```python
from build123d import *

# Parameters (mm, degrees)
SKETCH_1_R      = 3
EXTRUDE_1_DEPTH = 14
CHAMFER_1_SIZE  = 0.1


with BuildPart() as part:
    # 草图1 → 凸台-拉伸1 (new, symmetric)
    with BuildSketch(Plane(origin=(0, 0, 0), x_dir=(1, 0, 0), z_dir=(0, 1, 0))):
        with Locations(Location((0, 0, 0), (0, 0, 270))):
            Circle(SKETCH_1_R)
    extrude(amount=EXTRUDE_1_DEPTH, both=True)

    # 草图3 → M4 Tapped Hole1 (revolve, cut)
    with BuildSketch(Plane(origin=(0, 14, 0), x_dir=(0, 0, 1), z_dir=(1, 0, 0))):
        Polygon((0, 0), (0, 28), (1.675, 28), (1.65, 27.975), (1.65, 0.375), (2.025, 0), align=None)
    revolve(axis=Axis((0, 20.35, 0), (0, -1, 0)), mode=Mode.SUBTRACT)

    # 倒角1
    chamfer_1_edges = [part.edges().sort_by_distance(p)[0] for p in [
        (0, -14, -3),
        (0, 14, -3),
    ]]
    chamfer(chamfer_1_edges, length=CHAMFER_1_SIZE)


solid = part.part
```
Can you work these out from the model? Positions are in its coordinate system, mm. Give positions to 0.01 mm unless a question says otherwise; leave off trailing zeros. Write each loop counter-clockwise with the first axis right and the second up, starting at its lowest first coordinate (ties: lowest second). Pieces come first, ordered by that corner, then holes. Notation, with made-up numbers: (-27, 26) -> (20, 26) arc R21 cw to (20, 45) -> close; hole circle Ø6 at (66.25, 21.25). An arc over 180 degrees is marked (long way). Write item = value, one per line.
(1) I need wall thicknesses on probe 1 along X at (y, z) = (-2.25, 0); probe 2 along Z at (x, y) = (-0.65, -4); probe 3 along X at (y, z) = (7.75, 1.05). Which ranges of each line are inside material? Lowest first, please. Write a range as from..to.
Worked out:
probe_1 = -3..-1.65, 1.65..3
probe_2 = -2.93..-1.52, 1.52..2.93
probe_3 = -2.81..-1.27, 1.27..2.81
(2) I'm going to push flat-ended pins straight in: P1, Ø1.5, axis at y = 3.5, z = -1, coming from the -X side; P2, Ø3, axis at x = 0, z = 0.5, coming from the +Y side (3 decimals); P3, Ø3, axis at x = -2, y = 6, coming from the -Z side. Where does each tip first touch, or does it pass through?
Worked out:
P1 = -2.99
P2 = 13.975
P3 = -2.96
(3) Suppose I cut it at A-A on z = 0. Write out the boundary of the cut face in (x, y) (3 decimals), then the cut area to 3 significant figures.
Worked out:
outline = (-3, -13.9) -> (-2.9, -14) -> (-1.675, -14) -> (-1.65, -13.975) -> (-1.65, 13.625) -> (-2.025, 14) -> (-2.9, 14) -> (-3, 13.9) -> close; (1.65, -13.975) -> (1.675, -14) -> (2.9, -14) -> (3, -13.9) -> (3, 13.9) -> (2.9, 14) -> (2.025, 14) -> (1.65, 13.625) -> close
area = 75.4 mm^2
(4) Thinking about a two-plate mould opening in Z: for faces 1 (the face through (0.9, 0.19, 2.86)), 2 (the face through (-2, -14, 0)), 3 (the face through (-1.115, 0.018, -1.216)), which applies, released by +Z, released by -Z, zero draft, split by the parting line, or undercut?
Worked out:
face_1 = split by the parting line
face_2 = zero draft
face_3 = undercut
(5) Suppose I cut it at B-B on x = 0. Write out the boundary of the cut face in (y, z) (3 decimals).
Worked out:
outline = (-14, -2.9) -> (-13.9, -3) -> (13.9, -3) -> (14, -2.9) -> (14, -2.025) -> (13.625, -1.65) -> (-13.975, -1.65) -> (-14, -1.675) -> close; (-14, 1.675) -> (-13.975, 1.65) -> (13.625, 1.65) -> (14, 2.025) -> (14, 2.9) -> (13.9, 3) -> (-13.9, 3) -> (-14, 2.9) -> close
(6) Suppose I cut it at C-C on y = 1. Write out the boundary of the cut face in (x, z).
Worked out:
outline = circle Ø6 at (0, 0); hole circle Ø3.3 at (0, 0)
